Geometry check sheet. Reference: the model listing, model coordinates, mm. Give positions to 0.01 mm unless a question says otherwise; leave off trailing zeros. Order: outer loops, then holes, each group sorted by start corner. A loop starts at its lowest first (then second) coordinate and runs counter-clockwise, first axis right, second up. Notation, with made-up numbers: M 4.5,55.25 L 63.5,55.25 A29 cw 63.5,82.25 Z; hole C 30.25,34 d7. An arc over 180 degrees is marked long. Put each result on its own line as item: value. Start each with the question number.
Q1. Section check B-B on x = 10.5. Record the cut outline in (y, z), then the cut area to 3 significant figures.
Q2. Material ranges on L1, parallel to X at y = 1.85, z = 8; L2, parallel to X at y = 0.9, z = -29; L3, parallel to Z at x = 17.5, y = 1.6, recorded low to high.
Q3. Section check A-A on z = -1. Record the cut outline in (x, y).
Q4. Section check C-C on y = 1.75. State how many separate pieces and enclosed holes the cut face has, then the cut area to 3 significant figures.
```python
from build123d import *

# Parameters (mm, degrees)
SKETCH1_W               = 41.4
SKETCH1_H               = 108.224
SKETCH1_W_2             = 3
SKETCH1_H_2             = 20.4448
BOSS_EXTRUDE1_DEPTH     = 3
CUT_EXTRUDE1_DEPTH      = 1
CUT_EXTRUDE1_DEPTH_BACK = 4
FILLET1_R               = 2


with BuildPart() as part:
    # Sketch1 → Boss-Extrude1 (new body)
    with BuildSketch(Plane(origin=(0, 0, 0), x_dir=(1, 0, 0), z_dir=(0, 1, 0))):
        Rectangle(SKETCH1_W, SKETCH1_H)
        with Locations((16.2, 40.8896)):
            Rectangle(SKETCH1_W_2, SKETCH1_H_2, mode=Mode.SUBTRACT)
        with Locations((16.2, 0)):
            Rectangle(SKETCH1_W_2, SKETCH1_H_2, mode=Mode.SUBTRACT)
        with Locations((16.2, -40.8896)):
            Rectangle(SKETCH1_W_2, SKETCH1_H_2, mode=Mode.SUBTRACT)
        with Locations((-16.2, -40.8896)):
            Rectangle(SKETCH1_W_2, SKETCH1_H_2, mode=Mode.SUBTRACT)
        with Locations((-16.2, 0)):
            Rectangle(SKETCH1_W_2, SKETCH1_H_2, mode=Mode.SUBTRACT)
        with Locations((-16.2, 40.8896)):
            Rectangle(SKETCH1_W_2, SKETCH1_H_2, mode=Mode.SUBTRACT)
    extrude(amount=BOSS_EXTRUDE1_DEPTH)

    # Sketch2 → Cut-Extrude1 (cut, two sides)
    with BuildSketch(Plane(origin=(0, 3, 0), x_dir=(1, 0, 0), z_dir=(0, 1, 0))) as cut_extrude1_sk:
        Polygon((-5.35, 51.112), (-14.7, 51.112), (-14.7, 30.6672), (-14.7, 18.2224), (-5.35, 18.2224), align=None)
        Polygon((14.7, 51.112), (5.35, 51.112), (5.35, 18.2224), (14.7, 18.2224), (14.7, 30.6672), align=None)
    extrude(amount=CUT_EXTRUDE1_DEPTH, mode=Mode.SUBTRACT)
    extrude(cut_extrude1_sk.sketch, amount=-CUT_EXTRUDE1_DEPTH_BACK, mode=Mode.SUBTRACT)

    # Fillet1
    fillet1_edges = [part.edges().sort_by_distance(p)[0] for p in [
        (-5.35, 1.5, -18.2224),
        (-5.35, 1.5, -51.112),
        (5.35, 1.5, -18.2224),
        (5.35, 1.5, -51.112),
        (20.7, 1.5, 54.112),
        (-20.7, 1.5, 54.112),
        (-20.7, 1.5, -54.112),
        (20.7, 1.5, -54.112),
    ]]
    fillet(fillet1_edges, radius=FILLET1_R)


solid = part.part
```
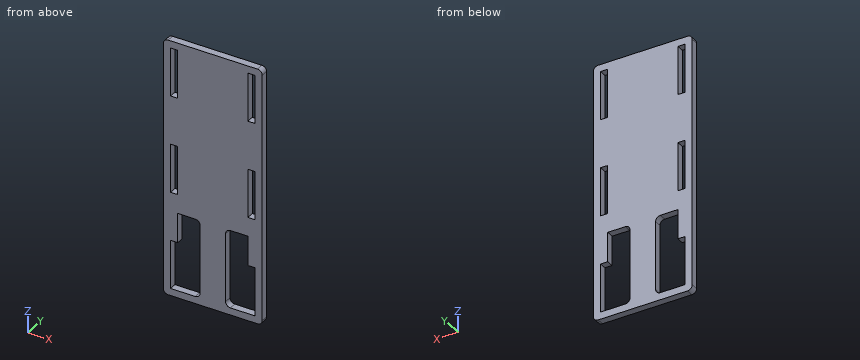
Results found:
1. outline: M 0,-54.11 L 3,-54.11 L 3,-51.11 L 0,-51.11 Z; M 0,-18.22 L 3,-18.22 L 3,54.11 L 0,54.11 Z
1. area: 226 mm^2
2. L1: x = -20.7 to -17.7, -14.7 to 14.7, 17.7 to 20.7
2. L2: x = -20.7 to -14.7, -5.35 to 5.35, 14.7 to 20.7
2. L3: z = -54.11 to -51.11, -30.67 to -10.22, 10.22 to 30.67, 51.11 to 54.11
3. outline: M -20.7,0 L -17.7,0 L -17.7,3 L -20.7,3 Z; M -14.7,0 L 14.7,0 L 14.7,3 L -14.7,3 Z; M 17.7,0 L 20.7,0 L 20.7,3 L 17.7,3 Z
4. separate pieces: 1
4. enclosed holes: 6
4. area: 3,500 mm^2
